Solid Edge part; units mm, degrees
sketch "Sketch1" plane through (0, 0, 0) normal (0, 0, 1) x (1, 0, 0)
  line L0 (-88.9, -31.75) -> (88.9, -31.75)
  line L1 (88.9, -31.75) -> (88.9, 31.75)
  line L2 (88.9, 31.75) -> (-88.9, 31.75)
  line L3 (-88.9, 31.75) -> (-88.9, -31.75)
extrude "Protrusion1" add sketch "Sketch1" along normal blind 50.8
sketch "Sketch2" plane through (0, -31.75, 25.4) normal (0, -1, 0) x (1, 0, 0)
  arc A0 (-88.9, 23.3785) -> (88.9, 23.3785) centre (0, -1930.4) cw
extrude "ExtrudedCutout_3" cut sketch "Sketch2" against normal blind 91.9194 material side at (0, -31.75, 50.85)
sketch "Sketch3" plane through (0, -31.75, 25.4) normal (0, -1, 0) x (1, 0, 0)
  arc A0 (88.9, -2.0481) -> (-88.9, -2.0481) centre (0, -1930.4) ccw
extrude "ExtrudedCutout_6" cut sketch "Sketch3" along normal mid plane 192.7852 material side at (0, -31.75, 25.45)
sketch "Sketch4" plane through (0, 31.75, 12.7) normal (0, 1, 0) x (1, 0, 0)
  line L0 (-88.9, 1.0241) -> (88.9, 1.0241)
extrude "ExtrudedCutout_7" cut sketch "Sketch4" along normal mid plane 206.9311 material side at (0, 31.75, 11.6259)
chamfer "Chamfer_4" distance 6.35 angle 45 4 edges at (0, 31.75, 11.6759) (-88.9, 0, 11.6759) (0, -31.75, 11.6759) (88.9, 0, 11.6759)
sketch "Sketch5" plane through (0, 0, 50.8) normal (0, 0, 1) x (0, 1, 0)
  circle A0 centre (0, 63.5) radius 12.7
  circle A1 centre (0, -63.5) radius 12.7
extrude "ExtrudedCutout_8" cut sketch "Sketch5" against normal blind 84.0346
Geometry check sheet. Reference: the model listing, model coordinates, mm. Round coordinates to 2 decimals unless told otherwise and drop trailing zeros. Order: outer loops, then holes, each group sorted by start corner. A loop starts at its lowest first (then second) coordinate and runs counter-clockwise, first axis right, second up. Notation, with made-up numbers: (45, 4.5) -> (58, 4.5) arc R26 ccw to (58, 38.5) -> close; hole circle Ø10 at (63.5, -30). An arc over 180 degrees is marked (long way). Return JSON: item names as keys, results as strings. Group by question number.
Q1. Section check C-C, the plane x = -63.5. Record the boundary of the cut face in (y, z), plus the area to 3 significant figures.
Q2. Section check A-A, the plane y = 0. Count the separate pieces of the cut face and the enclosed holes in it, plus the area to 3 significant figures.
Q3. Gauge pin test, flat end, axial feed: pin 1 (15 mm diameter, centred on x = -63.5, y = 0, fed in from +Z). Record the tip position at first contact, or that the pin passes through.
Q4. Release check for a two-part mould opening along Y. For faces 1 (the cylindrical face through (-51.1, -2.75, 18.3)), 2 (the flat face through (-88.9, 0, 21)), 3 (the flat face through (1, 31.75, 22)) record: released by +Y, released by -Y, zero draft, split by the parting line, or undercut.
Q5. Section check D-D, the plane z = 20.75. Record the boundary of the cut face in (x, y), plus the area to 3 significant figures.
Q6. Material ranges on probe 1 along X at (y, z) = (0, 18.5); probe 2 along X at (y, z) = (-5, 17.75); probe 3 along Y at (x, z) = (-63.5, 19.5), recorded low to high. Write a range as from..to.
Numbers:
{
 "1": {"outline": "(-31.75, 18.03) -> (-25.4, 11.68) -> (-12.7, 11.68) -> (-12.7, 24.36) -> (-31.75, 24.36) -> close; (12.7, 11.68) -> (25.4, 11.68) -> (31.75, 18.03) -> (31.75, 24.36) -> (12.7, 24.36) -> close", "area": "443 mm^2"},
 "2": {"separate pieces": "3", "enclosed holes": "0", "area": "1,640 mm^2"},
 "3": {"pin 1": "through"},
 "4": {"face 1": "undercut", "face 2": "zero draft", "face 3": "released by +Y"},
 "5": {"outline": "(-88.9, -31.75) -> (88.9, -31.75) -> (88.9, 31.75) -> (-88.9, 31.75) -> close; hole circle Ø25.4 at (-63.5, 0); hole circle Ø25.4 at (63.5, 0)", "area": "10,300 mm^2"},
 "6": {"probe 1": "-88.9..-76.2, -50.8..50.8, 76.2..88.9", "probe 2": "-88.62..-75.17, -51.83..51.83, 75.17..88.62", "probe 3": "-31.75..-12.7, 12.7..31.75"}
}
